from build123d import *

# Parameters (mm, degrees)
SKETCH_1_R               = 8.5
EXTRUDE_1_DEPTH          = 5
EXTRUDE_1_TAPER          = 4
SKETCH_3_R               = 5
CUT_EXTRUDE_1_DEPTH      = 1
SKETCH_4_R               = 6.6
CUT_EXTRUDE_2_DEPTH      = 2.5
CUT_EXTRUDE_3_DEPTH      = 13.278029158
CUT_EXTRUDE_3_DEPTH_BACK = 13.278029158
SKETCH_5_R               = 3


with BuildPart() as part:
    # Эскиз1 → Бобышка-Вытянуть1 (new body)
    with BuildSketch(Plane.XY):
        Circle(SKETCH_1_R)
    extrude(amount=EXTRUDE_1_DEPTH, taper=EXTRUDE_1_TAPER)

    # Эскиз3 → Вырез-Вытянуть1 (cut)
    with BuildSketch(Plane(origin=(0, 0, 0), x_dir=(-1, 0, 0), z_dir=(0, 0, -1))):
        Circle(SKETCH_3_R)
    extrude(amount=-CUT_EXTRUDE_1_DEPTH, mode=Mode.SUBTRACT)

    # Эскиз4 → Вырез-Вытянуть2 (cut)
    with BuildSketch(Plane.XY.offset(5)):
        Circle(SKETCH_4_R)
    extrude(amount=-CUT_EXTRUDE_2_DEPTH, mode=Mode.SUBTRACT)

    # Эскиз5 → Вырез-Вытянуть3 (cut, two sides: drawn at the far end of the back side and taken through both)
    with BuildSketch(Plane.XY.offset(2.5).offset(-CUT_EXTRUDE_3_DEPTH_BACK)):
        Circle(SKETCH_5_R)
    extrude(amount=CUT_EXTRUDE_3_DEPTH + CUT_EXTRUDE_3_DEPTH_BACK, mode=Mode.SUBTRACT)


solid = part.part
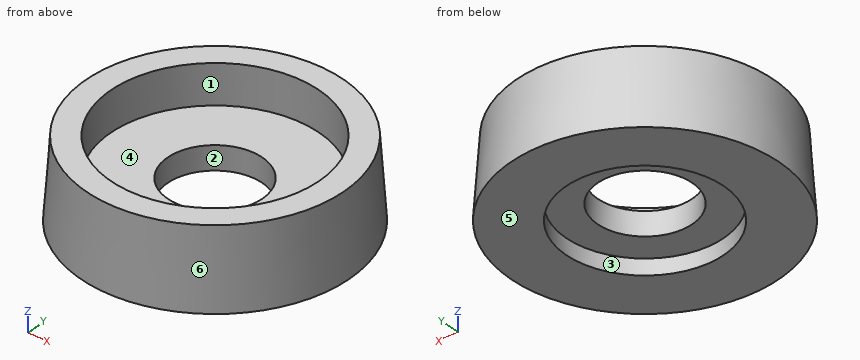
The model under review builds one solid part; all positions refer to its coordinate system, in mm. Face numbers are marked on the shaded views. A direction names the side the tool comes from. Give positions to 0.01 mm unless a question says otherwise; leave off trailing zeros. Loops run counter-clockwise (first coordinate to the right, second up) from the corner with the lowest first, then second, coordinate; pieces in that order, holes last. Notation, with made-up numbers: (44.25, -38.75) -> (54.25, -38.75) arc R30 ccw to (54.25, -7.75) -> close; hole circle Ø9 at (16, 77.25). An arc over 180 degrees is marked (long way). Put each result on its own line as item: value. Start each with the question number.
1. For the marked faces 1, 2 and 3, list the 3-axis set-ups (+Z, -Z, +X, -X, +Y, -Y) from which the entire face can be reached by the end or side of a thin tool; tool diameter is ignored.
2. We need section D-D on z = 4.65. State the section outline as (x, y) points, then the cut area to 3 significant figures.
3. Clearance check with flat-ended pins moving along their axes: P1, Ø9.5, axis at x = 0, y = 0, coming from the -Z side; P2, Ø2, axis at x = -0.5, y = 1.5, coming from the -Z side; P3, Ø2, axis at x = 5, y = 3.5, coming from the -Z side; P4, Ø3, axis at x = 6.5, z = 3.5, coming from the -Y side. State where each tip first meets the part, or that it passes through.
4. Mouldability with a two-part tool opening along X and no side actions: class the marked faces 4, 5 and 6 as released by +X, released by -X, zero draft, split by the parting line, or undercut.
5. We need section A-A on y = 0. State the section outline as (x, z) points.
6. We need section C-C on z = 1.6. State the section outline as (x, y) points, then the cut area to 3 significant figures.
7. Wall thickness on probe 1 along Z at (x, y) = (1, -4.5); probe 2 along Y at (x, z) = (5.25, 3.8); probe 3 along X at (y, z) = (0, 1.9): over which ranges is each line inside the solid? List them lowest first.
Determined:
1. face 1: +Z
1. face 2: +Z, -Z
1. face 3: -Z
2. outline: circle Ø16.35 at (0, 0); hole circle Ø13.2 at (0, 0)
2. area: 73.1 mm^2
3. P1: z = 1
3. P2: through
3. P3: z = 0
3. P4: y = -6.58
4. face 4: undercut
4. face 5: zero draft
4. face 6: split by the parting line
5. outline: (-8.5, 0) -> (-5, 0) -> (-5, 1) -> (-3, 1) -> (-3, 2.5) -> (-6.6, 2.5) -> (-6.6, 5) -> (-8.15, 5) -> close; (3, 1) -> (5, 1) -> (5, 0) -> (8.5, 0) -> (8.15, 5) -> (6.6, 5) -> (6.6, 2.5) -> (3, 2.5) -> close
6. outline: circle Ø16.78 at (0, 0); hole circle Ø6 at (0, 0)
6. area: 193 mm^2
7. probe 1: 1 to 2.5
7. probe 2: -6.34 to -4, 4 to 6.34
7. probe 3: -8.37 to -3, 3 to 8.37
